Work out the finished part from the listing and answer in its coordinate system (mm). A direction names the side the tool comes from. Coordinates: 2 decimals unless noted, no trailing zeros. Write each loop counter-clockwise with the first axis right and the second up, starting at its lowest first coordinate (ties: lowest second). Pieces come first, ordered by that corner, then holes. Notation, with made-up numbers: (80.25, 59.25) - (103.25, 59.25) arc R16 cw to (103.25, 78.25) - close; hole circle Ø1 at (76.5, 2.25). An arc over 180 degrees is marked (long way). Use a Markdown table: item, result. Add a question column.
(1) For a pull along Y with two mould halves and no side action, classify faces 3 (the face through (-29.43, -4.22, 67.44)), 4 (the face through (-29, -34, 71)), 5 (the face through (-29, 20, 71)), 6 (the face through (-16.639, -31.972, 89.536)) as released by +Y, released by -Y, zero draft, split by the parting line, or undercut.
(2) Find the intervals of material crossed by line 1 (Z direction, x = -29, y = 1); line 2 (Y direction, x = -24.5, z = 65.5); line 3 (X direction, y = 15, z = 71), in increasing order. Write a range as from..to.
(3) A tool of negligible diameter and unlimited length cuts with its end or side. For faces 1 (the face through (-29, -20, 66)), 2 (the face through (-24, -30, 61)), from which of +Z, -Z, +X, -X, +Y, -Y can it reach the whole face along a straight path? Write none if from no direction.
(4) The part is cut by section C-C, the plane z = 72.5. Give the vertices of the cut face in (x, y), then the cut area to 3 significant figures.
(5) Given pin 1 Ø1.5 at (y, z) = (4.5, 70) entering from +X; pin 2 Ø5 at (y, z) = (-26.5, 59) entering from -X; pin 3 Ø8 at (y, z) = (0, 74.5) entering from -X; pin 4 Ø5 at (x, y) = (-21, -2.5) entering from +Z, each flat-ended and moving along its own axis, determine where each tip first touches the part or whether it passes through.
(6) The part is cut by section A-A, the plane x = -24. Give the vertices of the cut face in (y, z).
(7) The part is cut by section B-B, the plane z = 65.5. Give the vertices of the cut face in (x, y), then the cut area to 3 significant figures.
(8) The part is cut by section D-D, the plane y = 16. Give the vertices of the cut face in (x, z), then the cut area to 3 significant figures.
from build123d import *

# Parameters (mm, degrees)
F0_R     = 3.2
F1_DEPTH = 20
F2_R     = 10
F3_DEPTH = 10
F4_R     = 22.5
F4_R_2   = 10
F5_DEPTH = 4
F6_R     = 10
F6_R_2   = 3.2
F7_DEPTH = 8


with BuildPart() as f1:
    # F0 (on Front) → F1 (new body, symmetric)
    with BuildSketch(Plane.XZ):
        with Locations((-28.7347137928, 70.5637484789)):
            Circle(F0_R)
    extrude(amount=F1_DEPTH, both=True)

    # F2 (on face) → F3 (join)
    with BuildSketch(Plane.XZ.offset(20)):
        with Locations((-28.7347137928, 70.5637484789)):
            Circle(F2_R)
    extrude(amount=F3_DEPTH)

    # F4 (on face) → F5 (join)
    with BuildSketch(Plane.XZ.offset(30)):
        with Locations((-28.7347137928, 70.5637484789)):
            Circle(F4_R)
        with Locations((-28.7347137928, 70.5637484789)):
            Circle(F4_R_2, mode=Mode.SUBTRACT)
        with Locations((-28.7347137928, 70.5637484789)):
            Circle(F4_R_2)
    extrude(amount=F5_DEPTH)

    # F6 (on face) → F7 (join)
    with BuildSketch(Plane(origin=(0, 20, 0), x_dir=(-1, 0, 0), z_dir=(0, 1, 0))):
        with Locations((28.7347137928, 70.5637484789)):
            Circle(F6_R)
        with Locations((28.7347137928, 70.5637484789)):
            Circle(F6_R_2, mode=Mode.SUBTRACT)
    extrude(amount=-F7_DEPTH)


solid = f1.part
Model answer:
| question | item | result |
|---|---|---|
| 1 | face 3 | undercut |
| 1 | face 4 | released by -Y |
| 1 | face 5 | released by +Y |
| 1 | face 6 | zero draft |
| 2 | line 1 | 67.37..73.75 |
| 2 | line 2 | -34..-20, 12..20 |
| 2 | line 3 | -38.73..-18.74 |
| 3 | face 1 | none |
| 3 | face 2 | +Y |
| 4 | outline | (-51.15, -34) - (-6.32, -34) - (-6.32, -30) - (-18.92, -30) - (-18.92, -20) - (-26.19, -20) - (-26.19, 12) - (-18.92, 12) - (-18.92, 20) - (-38.55, 20) - (-38.55, 12) - (-31.28, 12) - (-31.28, -20) - (-38.55, -20) - (-38.55, -30) - (-51.15, -30) - close |
| 4 | area | 696 mm^2 |
| 5 | pin 1 | x = -25.53 |
| 5 | pin 2 | x = -32.96 |
| 5 | pin 3 | x = -31.93 |
| 5 | pin 4 | through |
| 6 | outline | (-34, 48.57) - (-30, 48.57) - (-30, 61.76) - (-20, 61.76) - (-20, 79.37) - (-30, 79.37) - (-30, 92.56) - (-34, 92.56) - close; (12, 61.76) - (20, 61.76) - (20, 79.37) - (12, 79.37) - close |
| 7 | outline | (-50.66, -34) - (-6.81, -34) - (-6.81, -30) - (-20.11, -30) - (-20.11, -20) - (-37.36, -20) - (-37.36, -30) - (-50.66, -30) - close; (-37.36, 12) - (-20.11, 12) - (-20.11, 20) - (-37.36, 20) - close |
| 7 | area | 486 mm^2 |
| 8 | outline | circle Ø20 at (-28.73, 70.56) |
| 8 | area | 314 mm^2 |
